```python
from build123d import *

# Parameters (mm, degrees)
F1_DEPTH    = 5
F2_SIZE     = 3
F3_T1_DEPTH = 17.2474487139
F3_T3_DEPTH = 17.5


# Not quite as in the source:
# - a fillet or chamfer that OpenCascade refuses, or shapes differently, is made with other operations: its cross-section is extruded or revolved along the edge and cut away or added
# - a feature names something its author has since deleted; it is built from what else it names


with BuildPart() as f1:
    # F0 (on Top) → F1 (new body)
    with BuildSketch(Plane.XY):
        with BuildLine():
            Line((-13, 12), (-13, 0))
            Line((-13, 0), (-10, 0))
            Line((-10, 0), (-8, 0))
            Line((-8, 0), (-8, 5))
            Line((-8, 5), (-10, 5))
            Line((-10, 5), (-10, 12))
            Line((-10, 12), (-5, 12))
            Line((-5, 12), (-5, 15))
            ThreePointArc((-5, 15), (0, 16.7884008853), (5, 15))
            Line((5, 15), (5, 12))
            Line((5, 12), (10, 12))
            Line((10, 12), (10, 5))
            Line((10, 5), (8, 5))
            Line((8, 5), (8, 0))
            Line((8, 0), (10, 0))
            Line((10, 0), (13, 0))
            Line((13, 0), (13, 15))
            Line((13, 15), (10, 15))
            Line((10, 15), (8, 15))
            ThreePointArc((8, 15), (0, 18.8196946698), (-8, 15))
            Line((-8, 15), (-10, 15))
            Line((-10, 15), (-13, 15))
            Line((-13, 15), (-13, 12))
        make_face()
    extrude(amount=F1_DEPTH)

    # F2
    f2_edges = [f1.edges().sort_by_distance(p)[0] for p in [
        (-8, 0, 2.5),
        (8, 0, 2.5),
    ]]
    chamfer(f2_edges, length=F2_SIZE)

    # F3: fillet of radius 2.5 on 6 edges, made by hand

    # F3_s2 → F3_t1 (cut)
    with BuildSketch(Plane.XY.offset(-6.123724357)):
        with BuildLine():
            ThreePointArc((-11, 0), (-12.4364916731, 0.8683509127), (-13, 2.4494897428))
            Line((-13, 2.4494897428), (-13, 0))
            Line((-13, 0), (-11, 0))
        make_face()
        with BuildLine():
            ThreePointArc((13, 2.4494897428), (12.4364916731, 0.8683509127), (11, 0))
            Line((11, 0), (13, 0))
            Line((13, 0), (13, 2.4494897428))
        make_face()
    extrude(amount=F3_T1_DEPTH, mode=Mode.SUBTRACT)

    # F3_s4 → F3_t3 (cut)
    with BuildSketch(Plane.XY.offset(-6.25)):
        with BuildLine():
            ThreePointArc((-13, 12.5), (-12.267766953, 14.267766953), (-10.5, 15))
            Line((-10.5, 15), (-13, 15))
            Line((-13, 15), (-13, 12.5))
        make_face()
        with BuildLine():
            ThreePointArc((10.5, 15), (12.267766953, 14.267766953), (13, 12.5))
            Line((13, 12.5), (13, 15))
            Line((13, 15), (10.5, 15))
        make_face()
        with BuildLine():
            ThreePointArc((-7.5, 12), (-5.732233047, 12.732233047), (-5, 14.5))
            Line((-5, 14.5), (-5, 12))
            Line((-5, 12), (-7.5, 12))
        make_face()
        with BuildLine():
            ThreePointArc((5, 14.5), (5.732233047, 12.732233047), (7.5, 12))
            Line((7.5, 12), (5, 12))
            Line((5, 12), (5, 14.5))
        make_face()
    extrude(amount=F3_T3_DEPTH, mode=Mode.SUBTRACT)


solid = f1.part
```
Geometry check sheet. Reference: the model listing, model coordinates, mm. A direction names the side the tool comes from. Coordinates: 2 decimals unless noted, no trailing zeros. Loops run counter-clockwise (first coordinate to the right, second up) from the corner with the lowest first, then second, coordinate; pieces in that order, holes last.
Item 1: Thickness scan on line 1 (X direction, y = 10, z = 2.15); line 2 (X direction, y = 3.5, z = 2.9); line 3 (Y direction, x = -9.75, z = 1.5). Record the ranges inside material, lowest first.
Item 2: Sectioned sample at D-D, the plane x = -6.5. Record the boundary of the cut face in (y, z), then the cut area to 3 significant figures.
Item 3: Sectioned sample at C-C, the plane y = 16. Record the boundary of the cut face in (x, z), then the cut area to 3 significant figures.
Item 4: Go/stop test with flat-tipped pins: pin 1 Ø0.6 at (y, z) = (15, 1.5) entering from +X; pin 2 Ø1 at (x, z) = (9.5, 2) entering from +Y; pin 3 Ø3 at (x, z) = (8.5, 3.5) entering from -Y; pin 4 Ø10 at (x, y) = (-1, 3) entering from +Z. Record where each tip stops, or that it passes through.
Item 5: Sectioned sample at B-B, the plane z = 1.75. Record the boundary of the cut face in (x, y), then the cut area to 3 significant figures.
Item 6: Sectioned sample at A-A, the plane y = 7. Record the boundary of the cut face in (x, z).
Item 7: Release check for a two-part mould opening along Y. For faces 6 (the face through (-8, 4, 2)), 7 (the face through (5.713, 12.752, 2.465)), 8 (the face through (9, 12, 2)) record: released by +Y, released by -Y, zero draft, split by the parting line, or undercut.
Item 8: Access from +Z, -Z, +X, -X, +Y, -Y to the whole of each face (thin tool, end or side, straight path). Record for faces 1 (the face through (-9, 5, 2)), 2 (the face through (8, 4, 2)), 3 (the face through (-12.42, 0.85, 2.46)), 4 (the face through (-9, 15, 2)), 5 (the face through (9, 15, 2)).
Check result:
1. line 1: x = -13 to -10, 10 to 13
1. line 2: x = -13 to -8, 8 to 13
1. line 3: y = 1.25 to 5, 12 to 15
2. outline: (12.21, 0) - (16.51, 0) - (16.51, 5) - (12.21, 5) - close
2. area: 21.5 mm2
3. outline: (-7.08, 0) - (-3.44, 0) - (-3.44, 5) - (-7.08, 5) - close; (3.44, 0) - (7.08, 0) - (7.08, 5) - (3.44, 5) - close
3. area: 36.4 mm2
4. pin 1: stops at x = 11.69
4. pin 2: stops at y = 15
4. pin 3: stops at y = 1
4. pin 4: passes through
5. outline: (-13, 2.45) arc R2.5 ccw to (-11, 0) - (-8, 3) - (-8, 5) - (-10, 5) - (-10, 12) - (-7.5, 12) arc R2.5 ccw to (-5, 14.5) - (-5, 15) arc R7.88 cw to (5, 15) - (5, 14.5) arc R2.5 ccw to (7.5, 12) - (10, 12) - (10, 5) - (8, 5) - (8, 3) - (11, 0) arc R2.5 ccw to (13, 2.45) - (13, 12.5) arc R2.5 ccw to (10.5, 15) - (8, 15) arc R10.29 ccw to (-8, 15) - (-10.5, 15) arc R2.5 ccw to (-13, 12.5) - close
5. area: 153 mm2
6. outline: (-13, 0) - (-10, 0) - (-10, 5) - (-13, 5) - close; (10, 0) - (13, 0) - (13, 5) - (10, 5) - close
7. face 6: zero draft
7. face 7: released by -Y
7. face 8: undercut
8. face 1: +Z, -Z
8. face 2: +Z, -Z, -Y
8. face 3: +Z, -Z, -X, -Y
8. face 4: +Z, -Z, -X, +Y
8. face 5: +Z, -Z, +X, +Y
